from build123d import *

# Parameters (mm, degrees)
SKETCH_1_W                     = 22.5
SKETCH_1_H                     = 15
HOLE_WIZARD_M3_5_1_D           = 4.2
HOLE_WIZARD_M3_5_1_CBORE_D     = 7
HOLE_WIZARD_M3_5_1_CBORE_DEPTH = 3
HOLE_WIZARD_1_D                = 10.2
HOLE_WIZARD_1_CBORE_D          = 20.5
HOLE_WIZARD_1_CBORE_DEPTH      = 1
CHAMFER_1_SIZE                 = 0.2


with BuildPart() as part:
    # 草图1 → 旋转1 (revolve)
    with BuildSketch(Plane.XY, mode=Mode.PRIVATE) as revolve_1_sk:
        with Locations((11.25, 7.5)):
            Rectangle(SKETCH_1_W, SKETCH_1_H)
    revolve(revolve_1_sk.sketch.rotate(Axis((0, 15, 0), (0, -1, 0)), 270), axis=Axis((0, 15, 0), (0, -1, 0)))

    # M3.5 六角头机械螺钉的柱形沉头孔1 (through all)
    with Locations(Plane(origin=(0, 15, 0), x_dir=(1, 0, 0), z_dir=(0, 1, 0))):
        with Locations((14.722431864, 8.5), (14.722431864, -8.5), (0, -17), (-14.722431864, -8.5), (-14.722431864, 8.5), (0, 17)):
            CounterBoreHole(HOLE_WIZARD_M3_5_1_D / 2, HOLE_WIZARD_M3_5_1_CBORE_D / 2, HOLE_WIZARD_M3_5_1_CBORE_DEPTH)

    # 孔1 (through all)
    with Locations(Plane(origin=(0, 15, 0), x_dir=(1, 0, 0), z_dir=(0, 1, 0))):
        with Locations((0, 0)):
            CounterBoreHole(HOLE_WIZARD_1_D / 2, HOLE_WIZARD_1_CBORE_D / 2, HOLE_WIZARD_1_CBORE_DEPTH)

    # 倒角1
    chamfer_1_edges = [part.edges().sort_by_distance(p)[0] for p in [
        (-3.5, 15, -17),
        (-18.222431864, 15, -8.5),
        (-18.222431864, 15, 8.5),
        (-3.5, 15, 17),
        (11.222431864, 15, 8.5),
        (11.222431864, 15, -8.5),
        (0, 15, 22.5),
        (-10.25, 15, 0),
        (5.1, 14, 0),
    ]]
    chamfer(chamfer_1_edges, length=CHAMFER_1_SIZE)


solid = part.part
Source: CAD feature listing. Evaluate the final solid. Frame: model axes, mm. A direction names the side the tool comes from. Give positions to 0.01 mm unless a question says otherwise; leave off trailing zeros. Write each loop counter-clockwise with the first axis right and the second up, starting at its lowest first coordinate (ties: lowest second). Pieces come first, ordered by that corner, then holes. Notation, with made-up numbers: M 79.25,-8 L 106.25,-8 A20 ccw 106.25,7 Z; hole C -39.5,17.25 d10. An arc over 180 degrees is marked long. Answer as a JSON object with one key per item and string values.
Q1. Access query for faces 4 (the face through (16.337, 13.42, -5.395)), 5 (the face through (0.273, 5.916, 14.918)). Directions: +Z, -Z, +X, -X, +Y, -Y. A direction counts if a zero-diameter tool reaches every point of the face in a straight line with its end or side. Return the directions, or none.
Geometry check:
{"face 4": "+Y", "face 5": "+Y, -Y"}
Q2. Mould query, pull axis Z, two halves, no side actions, for faces 1 (the face through (5.3, 0, -0.3)), 2 (the face through (2, 12, 19)), 3 (the face through (-8.618, 7.504, -20.784)). Classes: +Z half, -Z half, draft (parallel to the pull), parting line (faces both ways), or undercut.
Geometry check:
{"face 1": "draft", "face 2": "undercut", "face 3": "parting line"}
Q3. Cut plane A-A, the plane y = 3.5. Return the cut outline in (x, z).
Geometry check:
{"outline": "C 0,0 d45; hole C -14.72,-8.5 d4.2; hole C -14.72,8.5 d4.2; hole C 0,0 d10.2; hole C 0,-17 d4.2; hole C 0,17 d4.2; hole C 14.72,-8.5 d4.2; hole C 14.72,8.5 d4.2"}
Q4. Cut plane B-B, the plane x = 0. Count the separate pieces of the cut face and the enclosed holes in it, then the cut area to 3 significant figures.
Geometry check:
{"separate pieces": "4", "enclosed holes": "0", "area": "369 mm^2"}
Q5. Contact query for flat-ended pins moving along their axis: P1, Ø2, axis at x = -13, z = 8.5, coming from the +Y side; P2, Ø1.5, axis at y = 11, z = -1.5, coming from the -X side; P3, Ø6.5, axis at x = 0, z = 17, coming from the -Y side; P4, Ø1.5, axis at y = 8.5, z = -5, coming from the -X side. Output: stop coordinate, or through.
Geometry check:
{"P1": "stops at y = 12", "P2": "stops at x = -22.49", "P3": "stops at y = 0", "P4": "stops at x = -22.09"}
Q6. Ray query, line 1 along X through (y, z) = (2.5, -8.5); line 2 along X through (y, z) = (8.5, -10); line 3 along Y through (x, z) = (-7, -2.5). Return the intervals inside material, ascending.
Geometry check:
{"line 1": "x = -20.83 to -16.82, -12.62 to 12.62, 16.82 to 20.83", "line 2": "x = -20.16 to -16.19, -13.25 to 13.25, 16.19 to 20.16", "line 3": "y = 0 to 14"}
